Autodesk Inventor part; units mm, degrees
ref_plane "YZ Plane" through (0, 0, 0) normal (1, 0, 0) x (0, 1, 0)
ref_plane "XZ Plane" through (0, 0, 0) normal (0, 1, 0) x (-1, 0, 0)
ref_plane "XY Plane" through (0, 0, 0) normal (0, 0, 1) x (1, 0, 0)
sketch "Sketch1" plane through (0, 0, 0) normal (0, 0, 1) x (1, 0, 0)
  line L0 (0, 0) -> (400, 0)
  line L1 (400, 0) -> (400, 200)
  line L2 (400, 200) -> (0, 200)
  line L3 (0, 200) -> (0, 0)
  line L4 (5, 5) -> (395, 5)
  line L5 (395, 5) -> (395, 195)
  line L6 (395, 195) -> (5, 195)
  line L7 (5, 195) -> (5, 5)
  dimension "d0" = 400
  dimension "d1" = 200
  dimension "d2" = 390
  dimension "d3" = 190
extrude "Extrusion1" add sketch "Sketch1" along normal blind 80
sketch "Sketch2" plane through (0, 0, 0) normal (0, -1, 0) x (1, 0, 0)
  line L0 (5, 0) -> (395, 0)
  line L1 (190, 0) -> (220, 0)
  line L2 (220, 0) -> (220, 10)
  line L3 (220, 10) -> (190, 10)
  line L4 (190, 10) -> (190, 0)
  point P0 (0, 0)
  dimension "d6" = 30
  dimension "d7" = 10
extrude "Extrusion2" cut sketch "Sketch2" against normal blind 80
sketch "Sketch3" plane through (0, 200, 0) normal (0, 1, 0) x (1, 0, 0)
  line L0 (190, -10) -> (220, -10)
  line L1 (190, 0) -> (5, 0)
  line L2 (220, -10) -> (190, -10)
  line L3 (190, -10) -> (190, 0)
  line L4 (190, 0) -> (220, 0)
  line L5 (220, 0) -> (220, -10)
  point P0 (0, 0)
extrude "Extrusion3" cut sketch "Sketch3" against normal blind 80
sketch "Sketch4" plane through (0, 0, 0) normal (0, 0, -1) x (-1, 0, 0)
  line L0 (-400, 200) -> (-220, 200)
  line L1 (0, 0) -> (-400, 0)
  line L2 (-400, 0) -> (-400, 200)
  line L3 (-400, 200) -> (0, 200)
  line L4 (0, 200) -> (0, 0)
extrude "Extrusion4" add sketch "Sketch4" along normal blind 5
sketch "Sketch5" plane through (0, 0, 80) normal (0, 0, 1) x (1, 0, 0)
  point P0 (0, 0)
properties part number "d"
Check sheet for the modelled part. Datum: model origin and axes. Units: mm. A direction names the side the tool comes from. Give positions to 0.01 mm unless a question says otherwise; leave off trailing zeros. Loops run counter-clockwise (first coordinate to the right, second up) from the corner with the lowest first, then second, coordinate; pieces in that order, holes last. Notation, with made-up numbers: M 44,15 L 96,15 A4 ccw 96,19 Z; hole C -27.75,-4 d4. An arc over 180 degrees is marked long. Use a Markdown table: item, result. Add a question column.
Q1. Tool access check on faces 1 (the flat face through (199, 4, 80)), 2 (the flat face through (203, 195, 39)). Record the directions out of +Z, -Z, +X, -X, +Y, -Y that give a thin tool (end or side, any length) a straight path to the whole face; none if there is none.
Q2. Mould release check, pull along X, two halves, no side actions. Record for faces 3 (the flat face through (203, 200, 38)), 4 (the flat face through (0, 101, 38)), 5 (the flat face through (5, 101, 39)), 6 (the flat face through (203, 101, 0)): pulls with the +X half, pulls with the -X half, needs draft (parallel to the pull), parting line crosses it, or undercut.
Q3. Sectioned sample at A-A, the plane y = 167.5. Record the cut outline in (x, z).
Q4. Go/stop test with a flat-tipped pin: pin 1 (1 mm diameter, centred on x = 156, y = 160, fed in from +Z). Record where the tip stops, or that it passes through.
Q5. Sectioned sample at B-B, the plane z = 69.5. Record the cut outline in (x, y).
Q6. Sectioned sample at C-C, the plane x = 259. Record the cut outline in (y, z).
Q7. Scan lines: line 1 along X through (y, z) = (54, 66.5); line 2 along Y through (x, z) = (333, 11.5); line 3 along Z through (x, y) = (66.5, 95). Record each from-to range of solid material in increasing order. Write a range as [from, to].
Verdict:
| question | item | result |
|---|---|---|
| 1 | face 1 | +Z, +X, -X, +Y, -Y |
| 1 | face 2 | +Z |
| 2 | face 3 | needs draft |
| 2 | face 4 | pulls with the -X half |
| 2 | face 5 | undercut |
| 2 | face 6 | undercut |
| 3 | outline | M 0,-5 L 400,-5 L 400,80 L 395,80 L 395,0 L 5,0 L 5,80 L 0,80 Z |
| 4 | pin 1 | z = 0 |
| 5 | outline | M 0,0 L 400,0 L 400,200 L 0,200 Z; hole M 5,5 L 395,5 L 395,195 L 5,195 Z |
| 6 | outline | M 0,-5 L 200,-5 L 200,80 L 195,80 L 195,0 L 5,0 L 5,80 L 0,80 Z |
| 7 | line 1 | [0, 5], [395, 400] |
| 7 | line 2 | [0, 5], [195, 200] |
| 7 | line 3 | [-5, 0] |
